Design review of the part built by this model. Coordinates are the model's own, in mm. Round coordinates to 2 decimals unless told otherwise and drop trailing zeros. Write each loop counter-clockwise with the first axis right and the second up, starting at its lowest first coordinate (ties: lowest second). Pieces come first, ordered by that corner, then holes. Notation, with made-up numbers: M -15.5,-36.75 L -7.5,-36.75 A23 ccw -7.5,-9.75 Z; hole C 61.5,81.25 d6. An arc over 180 degrees is marked long. One line per question, with ' | ' between items. Start each with the question number.
Item 1: Add section C-C, the plane y = 4.75. Give the number of separate pieces and of enclosed holes in the cut face, and give its area (3 significant figures).
Item 2: Add section A-A, the plane x = 47.5. State the section outline as (y, z) points, and give its area (3 significant figures).
Item 3: Add section D-D, the plane x = 210.5. State the section outline as (y, z) points.
Item 4: Insertion check: pin 1 Ø12 at (x, z) = (58.5, 78) entering from -Y; pin 2 Ø2 at (y, z) = (2.5, -13.5) entering from -X; pin 3 Ø2 at (y, z) = (2, -26) entering from -X; pin 4 Ø2 at (x, y) = (193, 2) entering from -Z. Each pin has a flat end and moves straight along its axis. Give the tip position at first contact, or say it passes through.
Item 5: For L1, parallel to Z at x = 34, y = 1.5; L2, parallel to X at y = 0.75, z = 34.5; L3, parallel to X at y = 4.75, z = -10, list the stretches that pass through material, from the lowest coordinate up.
Item 6: Add section B-B, the plane z = 3.5. State the section outline as (x, y) points.
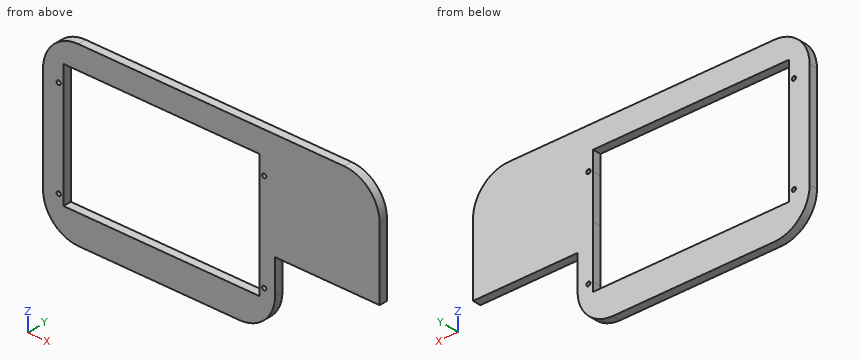
```python
from build123d import *

# Parameters (mm, degrees)
SKETCH1_R           = 1.75
BOSS_EXTRUDE1_DEPTH = 7


with BuildPart() as part:
    # Sketch1 → Boss-Extrude1 (new body)
    with BuildSketch(Plane(origin=(0, 0, 0), x_dir=(1, 0, 0), z_dir=(0, 1, 0))):
        with BuildLine():
            Line((117.322501745, 42.275563128), (-19.177498255, 42.275563128))
            ThreePointArc((-19.177498255, 42.275563128), (-40.39070169, 33.488766564), (-49.177498255, 12.275563128))
            Line((-49.177498255, 12.275563128), (-49.177498255, -76.986202657))
            ThreePointArc((-49.177498255, -76.986202657), (-40.39070169, -98.199406092), (-19.177498255, -106.986202657))
            Line((-19.177498255, -106.986202657), (156.322501745, -106.986202657))
            Line((156.322501745, -106.986202657), (205.849333343, -106.986202657))
            ThreePointArc((205.849333343, -106.986202657), (227.062536779, -98.199406092), (235.849333343, -76.986202657))
            Line((235.849333343, -76.986202657), (235.849333343, -16.324436872))
            Line((235.849333343, -16.324436872), (147.322501745, -16.324436872))
            Line((147.322501745, -16.324436872), (147.322501745, 12.275563128))
            ThreePointArc((147.322501745, 12.275563128), (138.535705181, 33.488766564), (117.322501745, 42.275563128))
        make_face()
        with Locations(Location((-35.865896123, -71.768154209, 0), (0, 0, 270))):
            Circle(SKETCH1_R, mode=Mode.SUBTRACT)
        Polygon((-31.865896123, -87.268154209), (-31.865896123, 17.731845791), (134.134103877, 17.731845791), (134.134103877, 10.231845791), (134.139344233, -34.268153014), (134.134104035, -71.167046413), (134.134103877, -71.16815413), (134.134103877, -87.268154209), align=None, mode=Mode.SUBTRACT)
        with Locations(Location((138.134103877, -72.683111915, 0), (0, 0, 270))):
            Circle(SKETCH1_R, mode=Mode.SUBTRACT)
        with Locations(Location((-35.865896123, 10.231845791, 0), (0, 0, 270))):
            Circle(SKETCH1_R, mode=Mode.SUBTRACT)
        with Locations(Location((138.134103877, 10.231845791, 0), (0, 0, 270))):
            Circle(SKETCH1_R, mode=Mode.SUBTRACT)
    extrude(amount=BOSS_EXTRUDE1_DEPTH)


solid = part.part
```
Computed values:
1) separate pieces: 1 | enclosed holes: 5 | area: 19,100 mm^2
2) outline: M 0,-42.28 L 7,-42.28 L 7,-17.73 L 0,-17.73 Z; M 0,87.27 L 7,87.27 L 7,106.99 L 0,106.99 Z | area: 310 mm^2
3) outline: M 0,16.32 L 7,16.32 L 7,106.62 L 0,106.62 Z
4) pin 1: passes through | pin 2: stops at x = -49.18 | pin 3: stops at x = -46.35 | pin 4: stops at z = 16.32
5) L1: z = -42.28 to -17.73, 87.27 to 106.99 | L2: x = -49.18 to -31.87, 134.14 to 235.85 | L3: x = -49.18 to -37.6, -34.13 to -31.87, 134.13 to 136.4, 139.87 to 147.32
6) outline: M -49.18,0 L -31.87,0 L -31.87,7 L -49.18,7 Z; M 134.14,0 L 147.32,0 L 147.32,7 L 134.14,7 Z
